```python
from build123d import *

# Parameters (mm, degrees)
ESQUISSE1_W = 4.5
ESQUISSE1_H = 5
CONG_1_R    = 0.5


with BuildPart() as part:
    # Esquisse1 → Révolution1 (revolve)
    with BuildSketch(Plane.XY, mode=Mode.PRIVATE) as r_volution1_sk:
        with Locations((4.25, 2.5)):
            Rectangle(ESQUISSE1_W, ESQUISSE1_H)
    revolve(r_volution1_sk.sketch.rotate(Axis((0, 0, 0), (0, 1, 0)), 90), axis=Axis((0, 0, 0), (0, 1, 0)))

    # Congé1
    cong_1_edges = [part.edges().sort_by_distance(p)[0] for p in [
        (0, 0, 2),
        (0, 0, 6.5),
        (0, 5, 6.5),
        (0, 5, 2),
    ]]
    fillet(cong_1_edges, radius=CONG_1_R)


solid = part.part
```
The model under review builds one solid part; all positions refer to its coordinate system, in mm. Coordinates: 2 decimals unless noted, no trailing zeros. Write each loop counter-clockwise with the first axis right and the second up, starting at its lowest first coordinate (ties: lowest second). Pieces come first, ordered by that corner, then holes. Notation, with made-up numbers: (51.25, 61.25) -> (108.25, 61.25) arc R21 cw to (108.25, 86.25) -> close; hole circle Ø9 at (-11.75, 60.5). An arc over 180 degrees is marked (long way). One line per item, written item: value. Start each with the question number.
Q1. To check wall thickness, follow probe 1 along X at (y, z) = (2.9, 0); probe 2 along Z at (x, y) = (-0.25, 1.8); probe 3 along Z at (x, y) = (0.5, 1.4). State the ranges of each line that lie inside material, in increasing order.
Q2. Add section A-A, the plane z = 0. Give the boundary of the cut face in (x, y).
Q3. Add section C-C, the plane y = 2.4. Give the boundary of the cut face in (x, z).
Q4. The part is to be moulded in two halves that separate along Z. For faces 1 (the face through (0, 0, 3)), 2 (the face through (3.955, 2.528, 5.158)), 3 (the face through (2, 3, 0)), say which applies: +Z half, -Z half, draft (parallel to the pull), parting line (faces both ways), or undercut.
Q5. Clearance check with a flat-ended pin moving along its axis: P1, Ø4.5, axis at x = 0, z = 0, coming from the +Y side. State where the tip first meets the part, or that it passes through.
Q6. Add section B-B, the plane x = 0. Give the boundary of the cut face in (y, z), then the cut area to 3 significant figures.
Response:
1. probe 1: -6.5 to -2, 2 to 6.5
1. probe 2: -6.5 to -1.98, 1.98 to 6.5
1. probe 3: -6.48 to -1.94, 1.94 to 6.48
2. outline: (-6.5, 0.5) arc R0.5 ccw to (-6, 0) -> (-2.5, 0) arc R0.5 ccw to (-2, 0.5) -> (-2, 4.5) arc R0.5 ccw to (-2.5, 5) -> (-6, 5) arc R0.5 ccw to (-6.5, 4.5) -> close; (2, 0.5) arc R0.5 ccw to (2.5, 0) -> (6, 0) arc R0.5 ccw to (6.5, 0.5) -> (6.5, 4.5) arc R0.5 ccw to (6, 5) -> (2.5, 5) arc R0.5 ccw to (2, 4.5) -> close
3. outline: circle Ø13 at (0, 0); hole circle Ø4 at (0, 0)
4. face 1: draft
4. face 2: parting line
4. face 3: undercut
5. P1: y = 4.93
6. outline: (0, -6) arc R0.5 ccw to (0.5, -6.5) -> (4.5, -6.5) arc R0.5 ccw to (5, -6) -> (5, -2.5) arc R0.5 ccw to (4.5, -2) -> (0.5, -2) arc R0.5 ccw to (0, -2.5) -> close; (0, 2.5) arc R0.5 ccw to (0.5, 2) -> (4.5, 2) arc R0.5 ccw to (5, 2.5) -> (5, 6) arc R0.5 ccw to (4.5, 6.5) -> (0.5, 6.5) arc R0.5 ccw to (0, 6) -> close
6. area: 44.6 mm²
